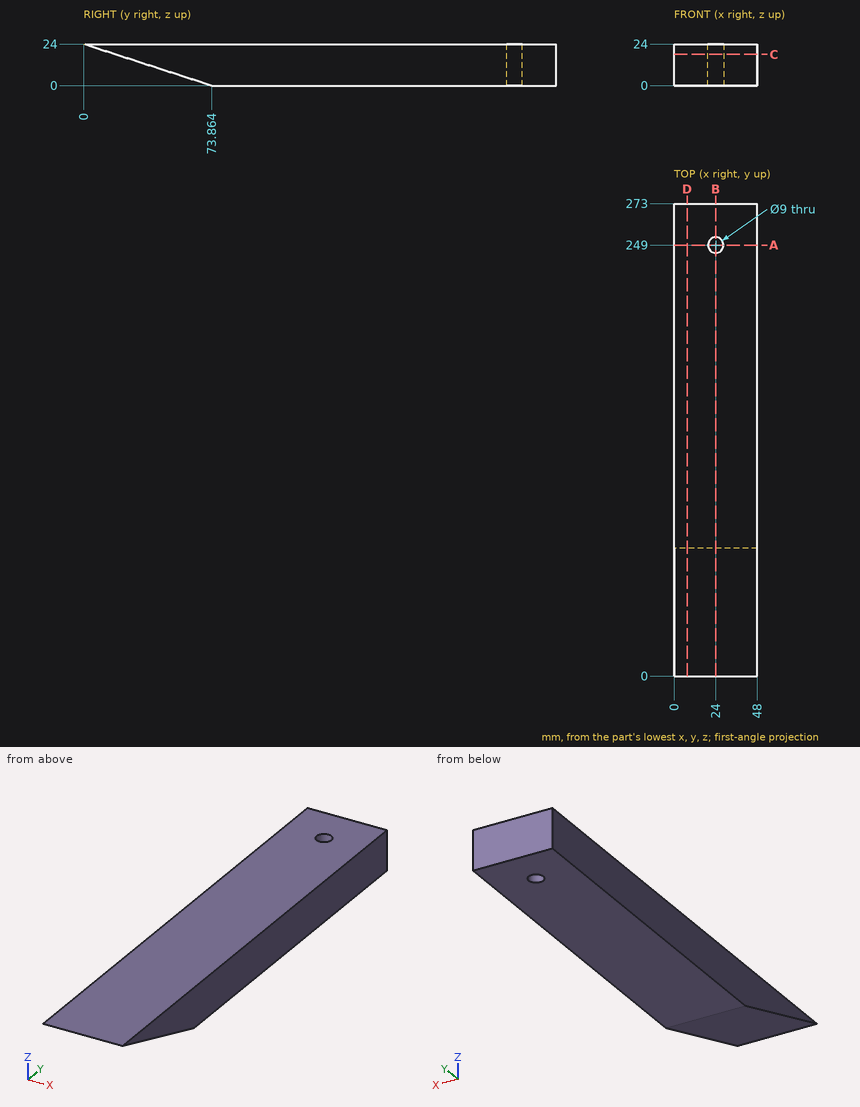
Study the drawing (mm; zero at the part's minimum x, y, z) and answer. Round coordinates to 2 decimals unless told otherwise and drop trailing zeros. Loops run counter-clockwise (first coordinate to the right, second up) from the corner with the lowest first, then second, coordinate; pieces in that order, holes last. Notation, with made-up numbers: (5, -12.75) -> (59, -12.75) arc R37 ccw to (59, 26.25) -> close; hole circle Ø8 at (31.5, 88). An arc over 180 degrees is marked (long way). One line per item, written item: value.
1) A cutting plane is placed at D-D (x = 7.5). Determine the outline of the cut face in (y, z) (1 decimal), and give its area (3 significant figures).
Answer list:
outline: (0, 24) -> (73.9, 0) -> (273, 0) -> (273, 24) -> close
area: 5,670 mm²
2) A cutting plane is placed at C-C (z = 18). Determine the outline of the cut face in (x, y), and give its area (3 significant figures).
Answer list:
outline: (0, 18.47) -> (48, 18.47) -> (48, 273) -> (0, 273) -> close; hole circle Ø9 at (24, 249)
area: 12,200 mm²
3) Consider L1, parallel to Z at x = 9.5, y = 53.5. Determine where the line is inside the solid, lowest interval first. Write a range as [from, to].
Answer list:
L1: z = [6.62, 24]
4) A cutting plane is placed at A-A (y = 249). Determine the outline of the cut face in (x, z).
Answer list:
outline: (0, 0) -> (19.5, 0) -> (19.5, 24) -> (0, 24) -> close; (28.5, 0) -> (48, 0) -> (48, 24) -> (28.5, 24) -> close
5) A cutting plane is placed at B-B (x = 24). Determine the outline of the cut face in (y, z) (1 decimal).
Answer list:
outline: (0, 24) -> (73.9, 0) -> (244.5, 0) -> (244.5, 24) -> close; (253.5, 0) -> (273, 0) -> (273, 24) -> (253.5, 24) -> close
